Can you work these out from the drawing? Everything is in mm from the part's minimum corner. A direction names the side the tool comes from. Coordinates: 2 decimals unless noted, no trailing zeros. Loops run counter-clockwise (first coordinate to the right, second up) from the corner with the lowest first, then second, coordinate; pieces in that order, holes last. Notation, with made-up numbers: M -12.5,19.5 L 1.5,19.5 A29 cw 1.5,45.5 Z; hole C 65,56.25 d11. An arc over 180 degrees is marked long. Use CSV: the item, a comma, the result in double quotes. Start each with the question number.
Q1. For pin 1 Ø4 at (x, y) = (31.5, 13) entering from -Z; pin 2 Ø1 at (y, z) = (41.5, 20) entering from +X; pin 3 Ø1.2 at (x, z) = (5.5, 21.5) entering from +Y; pin 4 Ø3 at (x, z) = (19.5, 23) entering from +Y, each with a flat end and sliding along its axis, tell me the tip position at first contact or that it passes through.
Q2. Please list where these lines run through material, in increasing order: probe 1 along X at (y, z) = (70.5, 22.1) (3 decimals); probe 2 along Y at (x, z) = (25, 35); probe 3 along Z at (x, y) = (22.5, 70). Write a range as [from, to].
Q3. If we section it at C-C (y = 10): Please give me the cut outline in (x, z).
Q4. If we section it at A-A (z = 22.1): Please give me the cut outline in (x, y) (3 decimals).
Q5. If we section it at B-B (x = 22.1): Please give me the cut outline in (y, z), and give its area (3 significant figures).
Q6. If we section it at D-D (z = 17): Please give me the cut outline in (x, y), and give its area (3 significant figures).
Q7. Which directions (+Z, -Z, +X, -X, +Y, -Y) give clear straight access to the entire face, cutting with the end or side of a thin tool? Please do the marked faces 1 and 2.
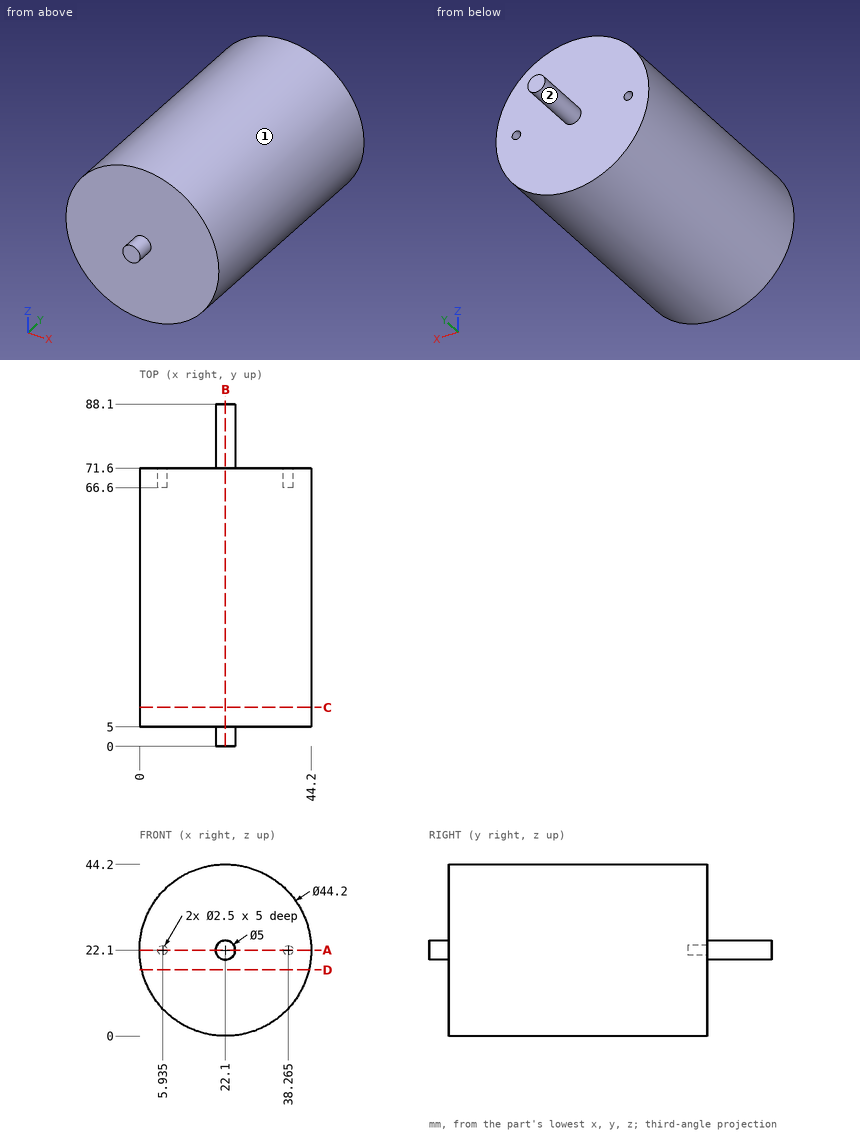
Results below:
1,pin 1,"z = 1.28"
1,pin 2,"x = 44.14"
1,pin 3,"y = 71.6"
1,pin 4,"y = 88.1"
2,probe 1,"[0, 4.685], [7.185, 37.015], [39.515, 44.2]"
2,probe 2,"[5, 71.6]"
2,probe 3,"[0, 44.2]"
3,outline,"C 22.1,22.1 d44.2"
4,outline,"M 0,5 L 19.6,5 L 19.6,0 L 24.6,0 L 24.6,5 L 44.2,5 L 44.2,71.6 L 39.515,71.6 L 39.515,66.6 L 37.015,66.6 L 37.015,71.6 L 24.6,71.6 L 24.6,88.1 L 19.6,88.1 L 19.6,71.6 L 7.185,71.6 L 7.185,66.6 L 4.685,66.6 L 4.685,71.6 L 0,71.6 Z"
5,outline,"M 0,19.6 L 5,19.6 L 5,0 L 71.6,0 L 71.6,19.6 L 88.1,19.6 L 88.1,24.6 L 71.6,24.6 L 71.6,44.2 L 5,44.2 L 5,24.6 L 0,24.6 Z"
5,area,"3,050 mm^2"
6,outline,"M 0.6,5 L 43.6,5 L 43.6,71.6 L 0.6,71.6 Z"
6,area,"2,860 mm^2"
7,face 1,"+Y, -Y"
7,face 2,"+Y"
